```python
from build123d import *

# Parameters (mm, degrees)
SKETCH_1_W          = 44.9
SKETCH_1_H          = 79.9
EXTRUDE_1_DEPTH     = 4
SKETCH_2_W          = 43.8
SKETCH_2_H          = 5.9
EXTRUDE_2_DEPTH     = 12.5
CUT_EXTRUDE_6_DEPTH = 52.15332345
SKETCH_7_R          = 1.75
CUT_EXTRUDE_7_DEPTH = 48.395642792
SKETCH_8_W          = 47.9
SKETCH_8_H          = 82.9
SKETCH_8_R          = 1.75
EXTRUDE_3_DEPTH     = 1.5
FILLET_1_R          = 1
SKETCH_9_R          = 7.5
CUT_EXTRUDE_8_DEPTH = 52.003588333
CHAMFER_1_SIZE      = 1.4
SKETCH_10_W         = 47.9
SKETCH_10_H         = 38.5
CUT_EXTRUDE_9_DEPTH = 2
SKETCH_11_R         = 9.5
SKETCH_11_R_2       = 7.5
EXTRUDE_1_2_DEPTH   = 2
EXTRUDE_1_2_DRAFT   = 1
SKETCH_12_R         = 9.5
EXTRUDE_4_DEPTH     = 2
FILLET_2_R          = 4
EXTRUDE_5_DEPTH     = 1.5
FILLET_3_R          = 1


with BuildPart() as part:
    # Эскиз1 → Extrude 1 (new body)
    with BuildSketch(Plane(origin=(0, 0, 0), x_dir=(1, 0, 0), z_dir=(0, 1, 0))):
        Rectangle(SKETCH_1_W, SKETCH_1_H)
    extrude(amount=EXTRUDE_1_DEPTH)

    # Эскиз2 → Бобышка-Вытянуть2 (add)
    with BuildSketch(Plane(origin=(0, 4, 0), x_dir=(1, 0, 0), z_dir=(0, 1, 0))):
        Rectangle(SKETCH_2_W, SKETCH_2_H)
    extrude(amount=EXTRUDE_2_DEPTH)

    # Эскиз3 → Вырез-Вытянуть6 (cut, through all)
    with BuildSketch(Plane.XY.offset(2.95)):
        with BuildLine():
            Line((-2.908454638, 16.097187923), (2.908454638, 16.097187923))
            ThreePointArc((2.908454638, 16.097187923), (11.009669484, 7.016387031), (21.505675783, 13.174672393))
            Line((21.505675783, 13.174672393), (23.649512702, 13.174672393))
            Line((23.649512702, 13.174672393), (22.1, 16.5))
            ThreePointArc((22.1, 16.5), (19.288225099, 23.288225099), (12.5, 26.1))
            Line((12.5, 26.1), (-12.5, 26.1))
            ThreePointArc((-12.5, 26.1), (-19.288225099, 23.288225099), (-22.1, 16.5))
            Line((-22.1, 16.5), (-23.550546649, 13.174672393))
            Line((-23.550546649, 13.174672393), (-21.505675783, 13.174672393))
            ThreePointArc((-21.505675783, 13.174672393), (-11.009669484, 7.016387031), (-2.908454638, 16.097187923))
        make_face()
    extrude(amount=-CUT_EXTRUDE_6_DEPTH, mode=Mode.SUBTRACT)

    # Эскиз7 → Вырез-Вытянуть7 (cut, through all)
    with BuildSketch(Plane(origin=(0, 4, 0), x_dir=(1, 0, 0), z_dir=(0, 1, 0))):
        with Locations(Location((0, -29.9, 0), (0, 0, 270))):
            Circle(SKETCH_7_R)
        with Locations(Location((0, 29.9, 0), (0, 0, 270))):
            Circle(SKETCH_7_R)
    extrude(amount=-CUT_EXTRUDE_7_DEPTH, mode=Mode.SUBTRACT)

    # Эскиз8 → Бобышка-Вытянуть3 (add)
    with BuildSketch(Plane.XZ):
        Rectangle(SKETCH_8_W, SKETCH_8_H)
        with Locations(Location((0, 29.9, 0), (0, 0, 90))):
            Circle(SKETCH_8_R, mode=Mode.SUBTRACT)
        with Locations(Location((0, -29.9, 0), (0, 0, 90))):
            Circle(SKETCH_8_R, mode=Mode.SUBTRACT)
    extrude(amount=EXTRUDE_3_DEPTH)

    # Скругление1
    fillet_1_edges = [part.edges().sort_by_distance(p)[0] for p in [
        (-23.95, -1.5, 0),
        (0, -1.5, -41.45),
        (23.95, -1.5, 0),
        (0, -1.5, 41.45),
    ]]
    fillet(fillet_1_edges, radius=FILLET_1_R)

    # Эскиз9 → Вырез-Вытянуть8 (cut, through all)
    with BuildSketch(Plane.XZ.offset(1.5)):
        with Locations(Location((0, 13.45, 0), (0, 0, 270))):
            Circle(SKETCH_9_R)
    extrude(amount=-CUT_EXTRUDE_8_DEPTH, mode=Mode.SUBTRACT)

    # Фаска1
    chamfer_1_edges = [part.edges().sort_by_distance(p)[0] for p in [
        (0, -1.5, 28.15),
        (0, -1.5, -31.65),
    ]]
    chamfer(chamfer_1_edges, length=CHAMFER_1_SIZE)

    # Эскиз10 → Вырез-Вытянуть9 (cut)
    with BuildSketch(Plane(origin=(0, 4, 0), x_dir=(1, 0, 0), z_dir=(0, 1, 0))):
        with Locations((0, 22.2)):
            Rectangle(SKETCH_10_W, SKETCH_10_H)
        with Locations((0, -22.2)):
            Rectangle(SKETCH_10_W, SKETCH_10_H)
    extrude(amount=-CUT_EXTRUDE_9_DEPTH, mode=Mode.SUBTRACT)


with BuildPart() as extrude_1_2_tool:
    # Эскиз11 → Extrude 1 2 (with draft: the straight prism first)
    with BuildSketch(Plane(origin=(0, 2, 0), x_dir=(1, 0, 0), z_dir=(0, 1, 0))):
        with Locations((0, -13.45)):
            Circle(SKETCH_11_R)
        with Locations((0, -13.45)):
            Circle(SKETCH_11_R_2, mode=Mode.SUBTRACT)
    extrude(amount=EXTRUDE_1_2_DEPTH)
    # Extrude 1 2: the draft: its side faces are tilted about the plane it starts from
    extrude_1_2_sides = [extrude_1_2_tool.faces().sort_by_distance(p)[0] for p in [
        (-9.5, 3, 13.45),
        (-7.5, 3, 13.45),
    ]]
    draft(extrude_1_2_sides, Plane(origin=(0, 2, 0), x_dir=(1, 0, 0), z_dir=(0, 1, 0)), EXTRUDE_1_2_DRAFT)


with BuildPart() as part_1:
    add(part.part)

    # Extrude 1 2: add extrude_1_2_tool
    add(extrude_1_2_tool.part)

    # Эскиз12 → Бобышка-Вытянуть4 (add)
    with BuildSketch(Plane(origin=(0, 4, 0), x_dir=(1, 0, 0), z_dir=(0, 1, 0))):
        with Locations(Location((0, -13.45, 0), (0, 0, 270))):
            Circle(SKETCH_12_R)
    extrude(amount=EXTRUDE_4_DEPTH)

    # Скругление2
    # the kernel refuses this fillet: 4 mm, written as the material it takes off along each edge
    with BuildSketch(Plane(origin=(0, 6, 13.45), x_dir=(0, 0, 1), z_dir=(-1, 0, 0))) as fillet_2_piece_1:
        with BuildLine():
            CenterArc((6.035898385, -4), FILLET_2_R, 30, 60)
            Line((6.035898385, 0), (6.035898385, 0.08))
            Line((6.035898385, 0.08), (9.5, 0.08))
            Line((9.5, 0.08), (9.58, 0))
            ThreePointArc((9.58, 0), (9.58, -1), (9.569282032, -1.96))
            Line((9.569282032, -1.96), (9.5, -2))
        make_face()
    revolve(axis=Axis((0, 6, 13.45), (0, 1, 0)), mode=Mode.SUBTRACT)
    # the kernel refuses this fillet: 4 mm, written as the material it takes off along each edge
    with BuildSketch(Plane(origin=(0, 2, 13.45), x_dir=(0.9999318130918542, 0, -0.011677720960747706), z_dir=(-0.011677720960747706, 0, -0.9999318130918542))) as fillet_2_2_piece_1:
        with BuildLine():
            CenterArc((7.5 + FILLET_2_R, FILLET_2_R * 0.00872686779076), FILLET_2_R, 180, 1)
            Line((7.5 + FILLET_2_R * 0.000152304843608, -FILLET_2_R * 0.00872553864652), (7.5 - FILLET_2_R * 0.0198446490595, -FILLET_2_R * 0.00907458677527))
            Line((7.5 - FILLET_2_R * 0.0198446490595, -FILLET_2_R * 0.00907458677527), (7.5 - FILLET_2_R * 0.02, -FILLET_2_R * 0.000174537355815))
            Line((7.5 - FILLET_2_R * 0.02, -FILLET_2_R * 0.000174537355815), (7.5 - FILLET_2_R * 0.02, FILLET_2_R * 0.00872686779076))
            Line((7.5 - FILLET_2_R * 0.02, FILLET_2_R * 0.00872686779076), (7.5, FILLET_2_R * 0.00872686779076))
        make_face()
    revolve(axis=Axis((0, 2, 13.45), (0, -1, 0)), revolution_arc=271.338198667, mode=Mode.SUBTRACT)
    # the kernel refuses this fillet: 4 mm, written as the material it adds along each edge
    with BuildSketch(Plane(origin=(0, 4, 13.45), x_dir=(1, 0, 0), z_dir=(0, 0, 1))) as fillet_2_3_piece_1_section:
        with BuildLine():
            CenterArc((3.5, -4), FILLET_2_R, 0, 90)
            Line((3.5, 0), (3.5, 0.4))
            Line((3.5, 0.4), (7.53491013, 0.4))
            Line((7.53491013, 0.4), (7.934849208, -0.006980963))
            ThreePointArc((7.934849208, -0.006980963), (7.9, -2.034907471), (7.9, -4))
            Line((7.9, -4), (7.5, -4))
        make_face()
    fillet_2_3_piece_1 = revolve(axis=Axis((0, 4, 13.45), (0, 1, 0)), mode=Mode.PRIVATE)
    fillet_2_3_piece_1 = split(fillet_2_3_piece_1, bisect_by=Plane(origin=(0, 4, 13.45), z_dir=(0.011677720960747706, 0, 0.9999318130918542)), keep=Keep.TOP, mode=Mode.PRIVATE)
    fillet_2_3_piece_1 = split(fillet_2_3_piece_1, bisect_by=Plane(origin=(0, 4, 13.45), z_dir=(0.9999318130918542, 0, 0.011677720960747469)), keep=Keep.TOP, mode=Mode.PRIVATE)
    add(fillet_2_3_piece_1)
    with BuildSketch(Plane(origin=(0, 4, 13.45), x_dir=(1, 0, 0), z_dir=(0, 0, 1))) as fillet_2_3_piece_2_section:
        with BuildLine():
            CenterArc((3.5, -4), FILLET_2_R, 0, 90)
            Line((3.5, 0), (3.5, 0.4))
            Line((3.5, 0.4), (7.53491013, 0.4))
            Line((7.53491013, 0.4), (7.934849208, -0.006980963))
            ThreePointArc((7.934849208, -0.006980963), (7.9, -2.034907471), (7.9, -4))
            Line((7.9, -4), (7.5, -4))
        make_face()
    fillet_2_3_piece_2 = revolve(axis=Axis((0, 4, 13.45), (0, 1, 0)), mode=Mode.PRIVATE)
    fillet_2_3_piece_2 = split(fillet_2_3_piece_2, bisect_by=Plane(origin=(0, 4, 13.45), z_dir=(-0.011677720960747706, 0, -0.9999318130918542)), keep=Keep.TOP, mode=Mode.PRIVATE)
    fillet_2_3_piece_2 = split(fillet_2_3_piece_2, bisect_by=Plane(origin=(0, 4, 13.45), z_dir=(0.9999318130918542, 0, 0.011677720960747469)), keep=Keep.TOP, mode=Mode.PRIVATE)
    add(fillet_2_3_piece_2)
    with BuildSketch(Plane(origin=(0, 4, 13.45), x_dir=(1, 0, 0), z_dir=(0, 0, 1))) as fillet_2_3_piece_3_section:
        with BuildLine():
            CenterArc((3.5, -4), FILLET_2_R, 0, 90)
            Line((3.5, 0), (3.5, 0.4))
            Line((3.5, 0.4), (7.53491013, 0.4))
            Line((7.53491013, 0.4), (7.934849208, -0.006980963))
            ThreePointArc((7.934849208, -0.006980963), (7.9, -2.034907471), (7.9, -4))
            Line((7.9, -4), (7.5, -4))
        make_face()
    fillet_2_3_piece_3 = revolve(axis=Axis((0, 4, 13.45), (0, 1, 0)), mode=Mode.PRIVATE)
    fillet_2_3_piece_3 = split(fillet_2_3_piece_3, bisect_by=Plane(origin=(0, 4, 13.45), z_dir=(0.011677720960747706, 0, 0.9999318130918542)), keep=Keep.TOP, mode=Mode.PRIVATE)
    fillet_2_3_piece_3 = split(fillet_2_3_piece_3, bisect_by=Plane(origin=(0, 4, 13.45), z_dir=(-0.9999318130918542, 0, -0.011677720960747469)), keep=Keep.TOP, mode=Mode.PRIVATE)
    add(fillet_2_3_piece_3)
    with BuildSketch(Plane(origin=(0, 4, 13.45), x_dir=(1, 0, 0), z_dir=(0, 0, 1))) as fillet_2_3_piece_4_section:
        with BuildLine():
            CenterArc((3.5, -4), FILLET_2_R, 0, 90)
            Line((3.5, 0), (3.5, 0.4))
            Line((3.5, 0.4), (7.53491013, 0.4))
            Line((7.53491013, 0.4), (7.934849208, -0.006980963))
            ThreePointArc((7.934849208, -0.006980963), (7.9, -2.034907471), (7.9, -4))
            Line((7.9, -4), (7.5, -4))
        make_face()
    fillet_2_3_piece_4 = revolve(axis=Axis((0, 4, 13.45), (0, 1, 0)), mode=Mode.PRIVATE)
    fillet_2_3_piece_4 = split(fillet_2_3_piece_4, bisect_by=Plane(origin=(0, 4, 13.45), z_dir=(-0.011677720960747706, 0, -0.9999318130918542)), keep=Keep.TOP, mode=Mode.PRIVATE)
    fillet_2_3_piece_4 = split(fillet_2_3_piece_4, bisect_by=Plane(origin=(0, 4, 13.45), z_dir=(-0.9999318130918542, 0, -0.011677720960747469)), keep=Keep.TOP, mode=Mode.PRIVATE)
    add(fillet_2_3_piece_4)

    # Эскиз13 → Бобышка-Вытянуть5 (add)
    with BuildSketch(Plane.XZ.offset(1.5)):
        with BuildLine():
            Line((-11, 20.95), (-11, 3.952706076))
            Line((-11, 3.952706076), (11, 3.952706076))
            Line((11, 3.952706076), (11, 20.95))
            ThreePointArc((11, 20.95), (0, 9.95), (-11, 20.95))
        make_face()
    extrude(amount=-EXTRUDE_5_DEPTH)

    # Скругление3
    # the kernel refuses this fillet: 1 mm, written as the material it takes off along each edge
    with BuildSketch(Plane(origin=(0, 0, 20.95), x_dir=(0.827668100134072, 0, -0.5612178864046082), z_dir=(0.5612178864046082, 0, 0.827668100134072))) as fillet_3_piece_1_section:
        with BuildLine():
            CenterArc((11 + FILLET_3_R, -FILLET_3_R), FILLET_3_R, 90, 90)
            Line((11 + FILLET_3_R, 0), (11, 0))
            Line((11, 0), (11, -FILLET_3_R))
        make_face()
    fillet_3_piece_1 = revolve(axis=Axis((0, 0, 20.95), (0, 1, 0)), revolution_arc=111.719870778, mode=Mode.PRIVATE)
    fillet_3_piece_1 = fillet_3_piece_1 & Plane(origin=(0, 0, 13.45), x_dir=(0, 0, -1), z_dir=(0, -1, 0)) * Cylinder(7.5, 49, mode=Mode.PRIVATE)
    add(fillet_3_piece_1, mode=Mode.SUBTRACT)


solid = part_1.part
```
Work out the finished part from the listing and answer in its coordinate system (mm). A direction names the side the tool comes from. Round coordinates to 2 decimals unless told otherwise and drop trailing zeros. Write each loop counter-clockwise with the first axis right and the second up, starting at its lowest first coordinate (ties: lowest second). Pieces come first, ordered by that corner, then holes.
1) A cutting plane is placed at A-A on z = 29.9. Determine the outline of the cut face in (x, y).
2) A cutting plane is placed at C-C on z = -4.5. Determine the outline of the cut face in (x, y), and give its area (3 significant figures).
3) Consider probe 1 along Y at (x, z) = (14.5, -13); probe 2 along X at (y, z) = (1.35, 29.9); probe 3 along X at (y, z) = (-1.05, 13.45). Determine where each line is inside the solid, lowest interval first.
4) A cutting plane is placed at D-D on x = 12.5. Determine the outline of the cut face in (y, z).
5) Which of the six approach directions +Z, -Z, +X, -X, +Y, -Y give full straight-line access (tool end or side, diameter ignored) to faces 1 (the face through (-22.45, 1, 1)), 2 (the face through (0, 6, 2.95)), 3 (the face through (0, 4, 13))?
6) A cutting plane is placed at B-B on y = 11. Determine the outline of the cut face in (x, z), and give its area (3 significant figures).
7) Determine the mould class of faces 4 (the face through (0, 6, 13)), 5 (the face through (-0.08, 0.96, 28.15)), 6 (the face through (0, 1, -39.95)) for opening direction Z: pulls with the +Z half, pulls with the -Z half, needs draft (parallel to the pull), parting line crosses it, or undercut.
8) Flat-ended cylindrical pins translate along their axes: P1, Ø1.5, axis at y = 11, z = 1.5, coming from the -X side; P2, Ø19.5, axis at x = 0, z = 13.45, coming from the -Y side; P3, Ø18.5, axis at x = -5.5, z = 25.5, coming from the +Y side; P4, Ø5, axis at x = 9.5, z = 17, coming from the +Y side. Find the tip coordinate at first contact, or state that the pin passes through.
Entries:
1. outline: (-23.95, -0.5) arc R1 ccw to (-22.95, -1.5) - (-3.15, -1.5) - (-1.75, -0.1) - (-1.75, 2) - (-22.45, 2) - (-22.45, 0) - (-23.95, 0) - close; (1.75, -0.1) - (3.15, -1.5) - (22.95, -1.5) arc R1 ccw to (23.95, -0.5) - (23.95, 0) - (22.45, 0) - (22.45, 2) - (1.75, 2) - close
2. outline: (-23.95, -0.5) arc R1 ccw to (-22.95, -1.5) - (22.95, -1.5) arc R1 ccw to (23.95, -0.5) - (23.95, 0) - (22.45, 0) - (22.45, 2) - (-22.45, 2) - (-22.45, 0) - (-23.95, 0) - close
2. area: 161 mm2
3. probe 1: y = -1.5 to 2
3. probe 2: x = -22.45 to -1.75, 1.75 to 22.45
3. probe 3: x = -23.79 to -7.5, 7.5 to 23.79
4. outline: (-1.5, -40.45) arc R1 ccw to (-0.5, -41.45) - (0, -41.45) - (0, -39.95) - (2, -39.95) - (2, -2.95) - (6.9, -2.95) - (6.9, 2.95) - (2, 2.95) - (2, 39.95) - (0, 39.95) - (0, 41.45) - (-0.5, 41.45) arc R1 ccw to (-1.5, 40.45) - close
5. face 1: +Z, -Z, -X, +Y
5. face 2: +X, -X, +Y
5. face 3: -Y
6. outline: (-21.9, -2.95) - (-20.37, -2.95) - (-20.37, 2.95) - (-21.9, 2.95) - close; (-4.63, -2.95) - (4.63, -2.95) - (4.63, 2.95) - (-4.63, 2.95) - close; (20.37, -2.95) - (21.9, -2.95) - (21.9, 2.95) - (20.37, 2.95) - close
6. area: 72.7 mm2
7. face 4: needs draft
7. face 5: undercut
7. face 6: pulls with the -Z half
8. P1: stops at x = -21.9
8. P2: stops at y = -1.5
8. P3: stops at y = 6
8. P4: stops at y = 5.66
